Autodesk Inventor part; units mm, degrees
ref_plane "YZ Plane" through (0, 0, 0) normal (1, 0, 0) x (0, 1, 0)
ref_plane "XZ Plane" through (0, 0, 0) normal (0, 1, 0) x (-1, 0, 0)
ref_plane "XY Plane" through (0, 0, 0) normal (0, 0, 1) x (1, 0, 0)
sketch "Sketch1" plane through (0, 0, 0) normal (0, 1, 0) x (-1, 0, 0)
  line L0 (0, 0) -> (21.3426, 0)
  line L1 (21.3426, 0) -> (21.3426, -8)
  line L2 (21.3426, -8) -> (0, -8)
  line L3 (0, -8) -> (-38.6574, -8)
  line L4 (-38.6574, -8) -> (-38.6574, 0)
  line L5 (-38.6574, 0) -> (0, 0)
  dimension "d2" = 8
  dimension "d3" = 60
  dimension "d13" = 8
extrude "Extrusion1" add sketch "Sketch1" along normal blind 50
sketch "Sketch3" plane through (0, 0, 0) normal (0, 0, 1) x (1, 0, 0)
  circle A0 centre (-0.8634, 20.189) radius 7.5
  line L0 (-17.3634, -0.311) -> (-21.3634, 3.689)
  line L1 (-17.3634, -0.311) -> (15.6366, -0.311)
  line L2 (19.6366, 3.689) -> (15.6366, -0.311)
  line L3 (19.6366, 3.689) -> (19.6366, 36.689)
  line L4 (15.6366, 40.689) -> (19.6366, 36.689)
  line L5 (15.6366, 40.689) -> (-17.3634, 40.689)
  line L6 (-21.3634, 36.689) -> (-17.3634, 40.689)
  line L7 (-21.3634, 36.689) -> (-21.3634, 3.689)
  circle A1 centre (-16.3634, 35.689) radius 1.5
  circle A2 centre (14.6366, 4.689) radius 1.5
  circle A3 centre (14.6366, 35.689) radius 1.5
  circle A4 centre (-16.3634, 4.689) radius 1.5
  circle A5 centre (33.6574, 10) radius 1.5
  circle A6 centre (33.6574, 19.5) radius 1.5
  line L8 (38.6574, 0) -> (38.6574, 50)
  line L9 (-21.3426, 0) -> (38.6574, 0)
  point P0 (0, 0)
  dimension "d6" = 5
  dimension "d7" = 5
  dimension "d8" = 3
  dimension "d9" = 3
  dimension "d11" = 9.5
  dimension "d12" = 10
extrude "Extrusion2" cut sketch "Sketch3" against normal blind 10 contours A0 | A1 | A2 | A3 | A4 | A5 | A6
fillet "Fillet1" radius 5 2 edges at (38.6574, 0, -4) (-21.3426, 0, -4)
sketch "Sketch4" plane through (0, 50, 0) normal (0, 1, 0) x (1, 0, 0)
  circle A0 centre (-11.3426, 2.5) radius 1.5
  circle A1 centre (8.6574, 2.5) radius 1.5
  circle A2 centre (28.6574, 2.5) radius 1.5
  circle A3 centre (-11.3426, 4) radius 1.5
  circle A4 centre (8.6574, 4) radius 1.5
  circle A5 centre (28.6574, 4) radius 1.5
  line L0 (-25.013, 4) -> (50.4038, 4)
  line L1 (-21.3426, 8) -> (-21.3426, 0)
  line L2 (-21.3426, 0) -> (38.6574, 0)
  point P0 (0, 0)
  dimension "d21" = 3
  dimension "d22" = 10
  dimension "d23" = 20
  dimension "d24" = 20
  dimension "d25" = 4
  dimension "d26" = 3
  dimension "d27" = 3
hole "Hole1" at (-11.3426, 50, -4) at (8.6574, 50, -4) at (28.6574, 50, -4) direction (0, -1, 0) diameter 2.459 depth 20 tip angle 118
properties part number "X-Axis_motor_plate"
Could you check a few things on this model? Use its own coordinates, in mm. A direction names the side the tool comes from. Round coordinates to 2 decimals unless told otherwise and drop trailing zeros. Order: outer loops, then holes, each group sorted by start corner. A loop starts at its lowest first (then second) coordinate and runs counter-clockwise, first axis right, second up. Notation, with made-up numbers: M 85,87.25 L 142,87.25 A9 ccw 142,103.25 Z; hole C -26,36.5 d3. An arc over 180 degrees is marked long. One line per question, with ' | ' between items. Start each with the question number.
(1) Please list where these lines run through material, in increasing order: line 1 along Y through (x, z) = (-15.5, -2); line 2 along Y through (x, z) = (35, -5.75); line 3 along X through (y, z) = (20.5, -3.5).
(2) Suppose I cut it at C-C on y = 19.5. List the corners of the cut face in (x, z) for me, then the cut area to 3 significant figures.
(3) Suppose I cut it at B-B on x = 2.5. List the corners of the cut face in (y, z) for me, then the cut area to 3 significant figures.
(4) For P1, Ø5, axis at x = 14.64, y = 4.69, coming from the +Z side; P2, Ø1.5, axis at x = 8.66, z = -4, coming from the +Y side; P3, Ø2, axis at x = -11.34, z = -4, coming from the +Y side, each with a flat end and sliding along its axis, tell me the tip position at first contact or that it passes through.
(5) For faces 4 (the face through (-19.839, 1.426, -4.056)), 5 (the face through (27.44, 39.86, -4.16)), which set-ups out of +Z, -Z, +X, -X, +Y, -Y let a thin tool reach every point of the face, with its end or its side?
(6) Thinking about a two-plate mould opening in Z: for faces 1 (the face through (38.657, 27, -4)), 2 (the face through (9, 25, 0)), 3 (the face through (-10.594, 39.86, -4.976)), which applies, +Z half, -Z half, draft (parallel to the pull), parting line (faces both ways), or undercut?
(7) Suppose I cut it at A-A on y = 10. List the corners of the cut face in (x, z) for me.
(8) Suppose I cut it at D-D on z = -1.25. List the corners of the cut face in (x, y) for me.
Geometry results:
1) line 1: 0 to 3.46, 5.92 to 34.46, 36.92 to 50 | line 2: 0.18 to 9.33, 10.67 to 18.83, 20.17 to 50 | line 3: -21.34 to -8.36, 6.63 to 32.54, 34.78 to 38.66
2) outline: M -21.34,-8 L -8.33,-8 L -8.33,0 L -21.34,0 Z; M 6.6,-8 L 32.16,-8 L 32.16,0 L 6.6,0 Z; M 35.16,-8 L 38.66,-8 L 38.66,0 L 35.16,0 Z | area: 337 mm²
3) outline: M 0,-8 L 13.49,-8 L 13.49,0 L 0,0 Z; M 26.89,-8 L 50,-8 L 50,0 L 26.89,0 Z | area: 293 mm²
4) P1: z = 0 | P2: y = 29.71 | P3: y = 29.86
5) face 4: +Z, -Z, -X, -Y | face 5: +Y
6) face 1: draft | face 2: +Z half | face 3: undercut
7) outline: M -21.34,-8 L 32.16,-8 L 32.16,0 L -21.34,0 Z; M 35.16,-8 L 38.66,-8 L 38.66,0 L 35.16,0 Z
8) outline: M -21.34,5 A5 ccw -16.34,0 L 33.66,0 A5 ccw 38.66,5 L 38.66,50 L -21.34,50 Z; hole C -16.36,4.69 d3; hole C -16.36,35.69 d3; hole C -0.86,20.19 d15; hole C 14.64,4.69 d3; hole C 14.64,35.69 d3; hole C 33.66,10 d3; hole C 33.66,19.5 d3
